Verification items for this drawing (mm, ordinates from the low corner). A direction names the side the tool comes from. Round coordinates to 2 decimals unless told otherwise and drop trailing zeros. Loops run counter-clockwise (first coordinate to the right, second up) from the corner with the lowest first, then second, coordinate; pieces in that order, holes last. Notation, with made-up numbers: M -2.5,-38 L 21.5,-38 A25 cw 21.5,-2 Z; hole C -17,9 d1. An arc over 180 degrees is marked long. Use one line per item in the form item = value. Start each with the question number.
1. Go/stop test with flat-tipped pins: pin 1 (3 mm diameter, centred on x = 3, y = 31.5, fed in from -Z); pin 2 (3 mm diameter, centred on x = 4, z = 5, fed in from +Y); pin 3 (1.9 mm diameter, centred on x = 5, y = 9, fed in from -Z). Record where each tip stops, or that it passes through.
2. Cross-section at B-B (z = 37). Record the boundary of the cut face in (x, y).
3. Cross-section at C-C (y = 30). Record the boundary of the cut face in (x, z), then the cut area to 3 significant figures.
4. Material ranges on line 1 (Z direction, x = 1.5, y = 19.5); line 2 (X direction, y = 30, z = 50); line 3 (X direction, y = 9, z = 10), recorded low to high.
5. Cross-section at A-A (y = 26). Record the boundary of the cut face in (x, z).
6. Set-up check for the marked faces 4, 5 and 6: record each of +Z, -Z, +X, -X, +Y, -Y from which the full face is reachable in a straight line by a thin tool's end or side.
7. Draft check along Z on the marked faces 1, 2 and 3. Enter one of: pulls with the +Z half, pulls with the -Z half, needs draft (parallel to the pull), parting line crosses it, or undercut.
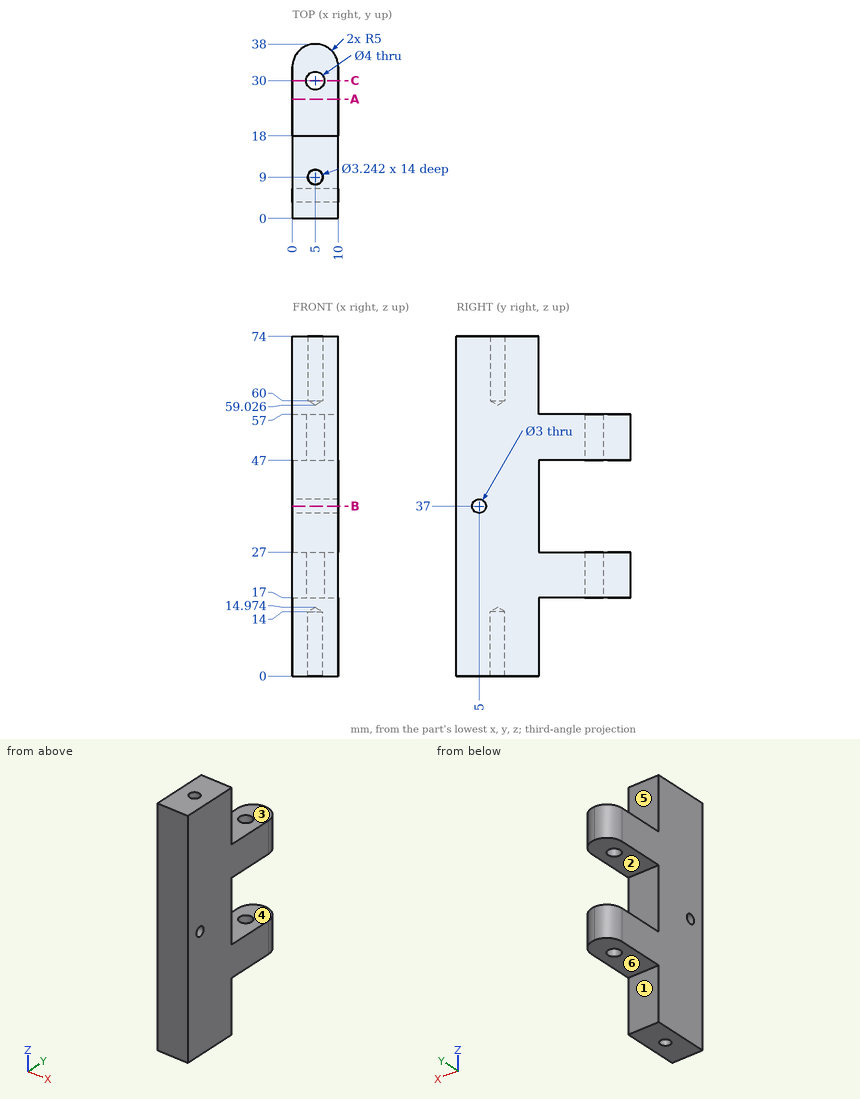
Reported:
q1.pin_1 = 17
q1.pin_2 = 18
q1.pin_3 = 14.4
q2.outline = M 0,0 L 10,0 L 10,3.5 L 0,3.5 Z; M 0,6.5 L 10,6.5 L 10,18 L 0,18 Z
q3.outline = M 0,17 L 3,17 L 3,27 L 0,27 Z; M 0,47 L 3,47 L 3,57 L 0,57 Z; M 7,17 L 10,17 L 10,27 L 7,27 Z; M 7,47 L 10,47 L 10,57 L 7,57 Z
q3.area = 120 mm²
q4.line_1 = 17 to 27, 47 to 57
q4.line_2 = 0 to 3, 7 to 10
q4.line_3 = 0 to 3.38, 6.62 to 10
q5.outline = M 0,17 L 10,17 L 10,27 L 0,27 Z; M 0,47 L 10,47 L 10,57 L 0,57 Z
q6.face_4 = +X, -X, +Y
q6.face_5 = +Z, +X, -X, +Y
q6.face_6 = -Z, +X, -X, +Y
q7.face_1 = needs draft
q7.face_2 = undercut
q7.face_3 = pulls with the +Z half
